from build123d import *

# Parameters (mm, degrees)
SKETCH1_W           = 1200
SKETCH1_H           = 1900
BOSS_EXTRUDE1_DEPTH = 5
CUT_EXTRUDE1_DEPTH  = 5
CUT_EXTRUDE2_DEPTH  = 3


with BuildPart() as part:
    # Sketch1 → Boss-Extrude1 (new body)
    with BuildSketch(Plane(origin=(0, 0, 0), x_dir=(1, 0, 0), z_dir=(0, 1, 0))):
        Rectangle(SKETCH1_W, SKETCH1_H)
    extrude(amount=BOSS_EXTRUDE1_DEPTH)

    # Sketch2 → Cut-Extrude1 (cut)
    with BuildSketch(Plane(origin=(0, 5, 0), x_dir=(1, 0, 0), z_dir=(0, 1, 0))):
        with BuildLine():
            Line((-500, 750), (-500, -750))
            ThreePointArc((-500, -750), (-502, -752), (-504, -750))
            Line((-504, -750), (-504, 750))
            ThreePointArc((-504, 750), (-502, 752), (-500, 750))
        make_face()
        with BuildLine():
            Line((-438, 750), (-438, -750))
            ThreePointArc((-438, -750), (-440, -752), (-442, -750))
            Line((-442, -750), (-442, 750))
            ThreePointArc((-442, 750), (-440, 752), (-438, 750))
        make_face()
        with BuildLine():
            Line((438, 750), (438, -750))
            ThreePointArc((438, -750), (440, -752), (442, -750))
            Line((442, -750), (442, 750))
            ThreePointArc((442, 750), (440, 752), (438, 750))
        make_face()
        with BuildLine():
            Line((500, 750), (500, -750))
            ThreePointArc((500, -750), (502, -752), (504, -750))
            Line((504, -750), (504, 750))
            ThreePointArc((504, 750), (502, 752), (500, 750))
        make_face()
    extrude(amount=-CUT_EXTRUDE1_DEPTH, mode=Mode.SUBTRACT)

    # Sketch4 → Cut-Extrude2 (cut)
    # profile 1 of 4: a face of its own
    with BuildSketch(Plane(origin=(0, 5, 0), x_dir=(1, 0, 0), z_dir=(0, 1, 0))):
        with BuildLine():
            Line((-435, -750), (-435, 750))
            ThreePointArc((-435, 750), (-440, 755), (-445, 750))
            Line((-445, 750), (-445, -750))
            ThreePointArc((-445, -750), (-440, -755), (-435, -750))
        make_face()
        with BuildLine():
            Line((-438, -750), (-438, 750))
            ThreePointArc((-438, 750), (-440, 752), (-442, 750))
            Line((-442, 750), (-442, -750))
            ThreePointArc((-442, -750), (-440, -752), (-438, -750))
        make_face(mode=Mode.SUBTRACT)
    # profile 2 of 4: a face of its own
    with BuildSketch(Plane(origin=(0, 5, 0), x_dir=(1, 0, 0), z_dir=(0, 1, 0))):
        with BuildLine():
            Line((-497, -750), (-497, 750))
            ThreePointArc((-497, 750), (-502, 755), (-507, 750))
            Line((-507, 750), (-507, -750))
            ThreePointArc((-507, -750), (-502, -755), (-497, -750))
        make_face()
        with BuildLine():
            Line((-500, -750), (-500, 750))
            ThreePointArc((-500, 750), (-502, 752), (-504, 750))
            Line((-504, 750), (-504, -750))
            ThreePointArc((-504, -750), (-502, -752), (-500, -750))
        make_face(mode=Mode.SUBTRACT)
    # profile 3 of 4: a face of its own
    with BuildSketch(Plane(origin=(0, 5, 0), x_dir=(1, 0, 0), z_dir=(0, 1, 0))):
        with BuildLine():
            Line((497, 750), (497, -750))
            ThreePointArc((497, -750), (502, -755), (507, -750))
            Line((507, -750), (507, 750))
            ThreePointArc((507, 750), (502, 755), (497, 750))
        make_face()
        with BuildLine():
            Line((500, 750), (500, -750))
            ThreePointArc((500, -750), (502, -752), (504, -750))
            Line((504, -750), (504, 750))
            ThreePointArc((504, 750), (502, 752), (500, 750))
        make_face(mode=Mode.SUBTRACT)
    # profile 4 of 4: a face of its own
    with BuildSketch(Plane(origin=(0, 5, 0), x_dir=(1, 0, 0), z_dir=(0, 1, 0))):
        with BuildLine():
            Line((435, 750), (435, -750))
            ThreePointArc((435, -750), (440, -755), (445, -750))
            Line((445, -750), (445, 750))
            ThreePointArc((445, 750), (440, 755), (435, 750))
        make_face()
        with BuildLine():
            Line((438, 750), (438, -750))
            ThreePointArc((438, -750), (440, -752), (442, -750))
            Line((442, -750), (442, 750))
            ThreePointArc((442, 750), (440, 752), (438, 750))
        make_face(mode=Mode.SUBTRACT)
    extrude(amount=-CUT_EXTRUDE2_DEPTH, mode=Mode.SUBTRACT)


solid = part.part
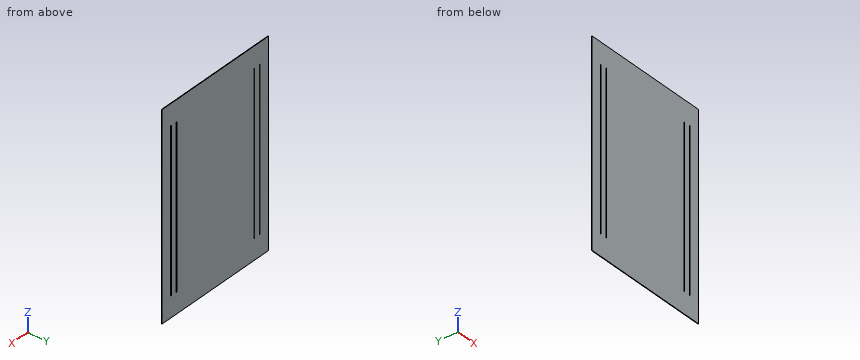
Design review of the part built by this model. Coordinates are the model's own, in mm. Coordinates: 2 decimals unless noted, no trailing zeros. Loops run counter-clockwise (first coordinate to the right, second up) from the corner with the lowest first, then second, coordinate; pieces in that order, holes last.
Item 1: Clearance check with a flat-ended pin moving along its axis: pin 1 (3 mm diameter, centred on x = 441.5, z = 118.5, fed in from +Y). State where the tip first meets the part, or that it passes through.
Completed:
pin 1: stops at y = 2
Item 2: Wall thickness on L1, parallel to X at y = 4.55, z = 447; L2, parallel to X at y = 1.95, z = -188: over which ranges is each line inside the solid? List them lowest first.
Completed:
L1: x = -600 to -507, -497 to -445, -435 to 435, 445 to 497, 507 to 600
L2: x = -600 to -504, -500 to -442, -438 to 438, 442 to 500, 504 to 600
Item 3: Add section B-B (z = -5). Give the number of separate pieces and of enclosed holes in the cut face, and give its area (3 significant figures).
Completed:
separate pieces: 5
enclosed holes: 0
area: 5,850 mm2
Item 4: Add section A-A (y = 4.05). Write out the cut boundary in (x, z), and give its area (3 significant figures).
Completed:
outline: (-600, -950) - (600, -950) - (600, 950) - (-600, 950) - close; hole (-507, -750) arc R5 ccw to (-497, -750) - (-497, 750) arc R5 ccw to (-507, 750) - close; hole (-445, -750) arc R5 ccw to (-435, -750) - (-435, 750) arc R5 ccw to (-445, 750) - close; hole (435, -750) arc R5 ccw to (445, -750) - (445, 750) arc R5 ccw to (435, 750) - close; hole (497, -750) arc R5 ccw to (507, -750) - (507, 750) arc R5 ccw to (497, 750) - close
area: 2,220,000 mm2
